Geometry: final body of the model. Coordinates: model frame, mm. A direction names the side the tool comes from. Coordinates: 2 decimals unless noted, no trailing zeros. Order: outer loops, then holes, each group sorted by start corner. A loop starts at its lowest first (then second) coordinate and runs counter-clockwise, first axis right, second up. Notation, with made-up numbers: (34, -11.75) -> (59, -11.75) arc R4 ccw to (59, -4.75) -> close; hole circle Ø7 at (41, 65.25). An arc over 180 degrees is marked (long way). Answer in a Markdown table with one row per item. Add a question column.
1) Section query B-B on z = -1. Return the cut outline in (x, y), then the cut area to 3 significant figures.
2) Section query A-A on z = -4. Return the cut outline in (x, y).
3) Section query C-C on x = -43. Return the cut outline in (y, z).
4) Set-up query: faces 5 (the face through (0, -12, -2)), 6 (the face through (-7, 13, -5)), 7 (the face through (-10, -6, -2)). Return all of +Z, -Z, +X, -X, +Y, -Y with unobstructed straight access to the full face (end or side cutting, diameter ignored); none if empty.
5) Ray query, line 1 (Y direction, x = 0, z = 0.45); line 2 (Z direction, x = -13.5, y = 5.5); line 3 (Z direction, x = -47, y = 36). Return the intervals inside material, ascending. Write a range as from..to.
6) Section query D-D on y = 23.5. Return the cut outline in (x, z).
7) Pull-direction query (Y, two-part tool) for faces 1 (the face through (-1.73, -7.81, -2.54)), 2 (the face through (-48, 34.2, -9)), 3 (the face through (-40, 28, -9)), 4 (the face through (3.4, -3.4, 0)); classes: +Y half, -Y half, draft (parallel to the pull), parting line (faces both ways), or undercut.
8) Contact query for flat-ended pins moving along their axis: P1, Ø6, axis at y = 17.5, z = -7.5, coming from the +X side; P2, Ø4, axis at y = 25, z = -3.5, coming from the -X side; P3, Ø1.8, axis at y = -5, z = -2.5, coming from the -X side. Output: stop coordinate, or through.
```python
from build123d import *

# Parameters (mm, degrees)
SKETCH1_R               = 10
SKETCH1_R_2             = 8
SKETCH1_R_3             = 4.5
BOSS_EXTRUDE1_DEPTH     = 1
BOSS_EXTRUDE2_START     = -5
SKETCH1_4_R             = 10
SKETCH1_4_R_2           = 8
BOSS_EXTRUDE2_DEPTH     = 5
BOSS_EXTRUDE3_START     = -6
BOSS_EXTRUDE3_DEPTH     = 6
BOSS_EXTRUDE4_DEPTH     = 5
BOSS_EXTRUDE5_REACH     = 76.3
SKETCH4_R               = 2
CUT_EXTRUDE1_DEPTH      = 78.507677039
CUT_EXTRUDE2_DEPTH      = 71.438909702
CUT_EXTRUDE2_DEPTH_BACK = 71.438909702


with BuildPart() as part:
    # Sketch1 → Boss-Extrude1 (new body)
    # profile 1 of 2: a face of its own
    with BuildSketch(Plane.XY):
        Circle(SKETCH1_R)
        Circle(SKETCH1_R_2, mode=Mode.SUBTRACT)
    # profile 2 of 2: a face of its own
    with BuildSketch(Plane.XY):
        Circle(SKETCH1_R_2)
        Circle(SKETCH1_R_3, mode=Mode.SUBTRACT)
    extrude(amount=BOSS_EXTRUDE1_DEPTH)

    # Sketch1<4> → Boss-Extrude2 (add)
    with BuildSketch(Plane.XY.offset(BOSS_EXTRUDE2_START)):
        Circle(SKETCH1_4_R)
        Circle(SKETCH1_4_R_2, mode=Mode.SUBTRACT)
    extrude(amount=BOSS_EXTRUDE2_DEPTH)

    # Sketch2 → Boss-Extrude3 (add)
    with BuildSketch(Plane.XY.offset(1).offset(BOSS_EXTRUDE3_START)):
        with BuildLine():
            Line((-40, 34.2), (-40, 22.5))
            Line((-40, 22.5), (-10, 0))
            ThreePointArc((-10, 0), (0, 10), (10, 0))
            Line((10, 0), (10, 34.2))
            Line((10, 34.2), (-40, 34.2))
        make_face()
        with BuildLine():
            ThreePointArc((10, 0), (0, -10), (-10, 0))
            Line((-10, 0), (-10, -12))
            Line((-10, -12), (10, -12))
            Line((10, -12), (10, 0))
        make_face()
    extrude(amount=BOSS_EXTRUDE3_DEPTH)

    # Sketch3 → Boss-Extrude4 (add)
    with BuildSketch(Plane(origin=(0, 34.2, 0), x_dir=(1, 0, 0), z_dir=(0, 1, 0))):
        Polygon((-55, -1), (-40, -1), (-40, 5), (-40, 19), (-55, 19), align=None)
        Polygon((-40, 19), (-40, 5), (-35, 5), (-35, 14.33), (-35, 19), align=None)
        Polygon((-35, 14.33), (-35, 5), (-25, 5), align=None)
        Polygon((-40, 5), (-40, -1), (10, -1), (10, 5), (-25, 5), (-35, 5), align=None)
    extrude(amount=BOSS_EXTRUDE4_DEPTH)

    # Boss-Extrude5: up to this plane
    boss_extrude5_end = Plane(origin=(-3.6, -4.8, -65.577553599), z_dir=(-0.6000000000000177, -0.7999999999999867, 0))
    # Sketch3<4> → Boss-Extrude5 (add, up to the surface)
    with BuildSketch(Plane(origin=(0, 34.2, 0), x_dir=(1, 0, 0), z_dir=(0, 1, 0)), mode=Mode.PRIVATE) as boss_extrude5_sk1:
        Polygon((-40, 19), (-40, 5), (-35, 5), (-35, 14.33), (-35, 19), align=None)
    boss_extrude5_tool1 = split(extrude(boss_extrude5_sk1.sketch, amount=-BOSS_EXTRUDE5_REACH, mode=Mode.PRIVATE), bisect_by=boss_extrude5_end, keep=Keep.BOTH, mode=Mode.PRIVATE)
    add(boss_extrude5_tool1.solids().sort_by_distance((-37.5, 34.2, -12))[0])
    # Sketch3<4> → Boss-Extrude5 (add, up to the surface)
    with BuildSketch(Plane(origin=(0, 34.2, 0), x_dir=(1, 0, 0), z_dir=(0, 1, 0)), mode=Mode.PRIVATE) as boss_extrude5_sk2:
        Polygon((-35, 14.33), (-35, 5), (-25, 5), align=None)
    boss_extrude5_tool2 = split(extrude(boss_extrude5_sk2.sketch, amount=-BOSS_EXTRUDE5_REACH, mode=Mode.PRIVATE), bisect_by=boss_extrude5_end, keep=Keep.BOTH, mode=Mode.PRIVATE)
    add(boss_extrude5_tool2.solids().sort_by_distance((-31.666667, 34.2, -8.11))[0])

    # Sketch4 → Cut-Extrude1 (cut, through all)
    with BuildSketch(Plane(origin=(0, 39.2, 0), x_dir=(1, 0, 0), z_dir=(0, 1, 0))):
        with Locations(Location((-47.5, 14, 0), (0, 0, 270))):
            Circle(SKETCH4_R)
        with Locations(Location((-47.5, 4, 0), (0, 0, 270))):
            Circle(SKETCH4_R)
    extrude(amount=-CUT_EXTRUDE1_DEPTH, mode=Mode.SUBTRACT)

    # Sketch5 → Cut-Extrude2 (cut, two sides: drawn at the far end of the back side and taken through both)
    with BuildSketch(Plane.XY.offset(1).offset(-CUT_EXTRUDE2_DEPTH_BACK)):
        Polygon((0, 20.48842356), (-24.948768587, 39.2), (10, 39.2), (10, 12.98842356), align=None)
    extrude(amount=CUT_EXTRUDE2_DEPTH + CUT_EXTRUDE2_DEPTH_BACK, mode=Mode.SUBTRACT)


solid = part.part
```
Result:
| question | item | result |
|---|---|---|
| 1 | outline | (-55, 34.2) -> (-40, 34.2) -> (-40, 22.5) -> (-10, 0) -> (-10, -12) -> (10, -12) -> (10, 12.99) -> (-24.95, 39.2) -> (-55, 39.2) -> close; hole circle Ø16 at (0, 0) |
| 1 | area | 1,280 mm2 |
| 2 | outline | (-55, 34.2) -> (-49.5, 34.2) -> (-49.5, 39.2) -> (-55, 39.2) -> close; (-45.5, 34.2) -> (-40, 34.2) -> (-40, 22.5) -> (-10, 0) -> (-10, -12) -> (10, -12) -> (10, 12.99) -> (-24.95, 39.2) -> (-45.5, 39.2) -> close; hole circle Ø16 at (0, 0) |
| 3 | outline | (34.2, -19) -> (39.2, -19) -> (39.2, 1) -> (34.2, 1) -> close |
| 4 | face 5 | +Z, -Z, +X, -X, -Y |
| 4 | face 6 | -Z, +X, +Y, -Y |
| 4 | face 7 | +Z, -Z, -X, -Y |
| 5 | line 1 | -12..-4.5, 4.5..20.49 |
| 5 | line 2 | -5..1 |
| 5 | line 3 | -19..-15.94, -12.06..-5.94, -2.06..1 |
| 6 | outline | (-40, -19) -> (-35, -19) -> (-35, -14.33) -> (-25, -5) -> (-4.02, -5) -> (-4.02, 1) -> (-40, 1) -> close |
| 7 | face 1 | undercut |
| 7 | face 2 | -Y half |
| 7 | face 3 | draft |
| 7 | face 4 | undercut |
| 8 | P1 | x = 6.2 |
| 8 | P2 | x = -40 |
| 8 | P3 | x = -10 |
